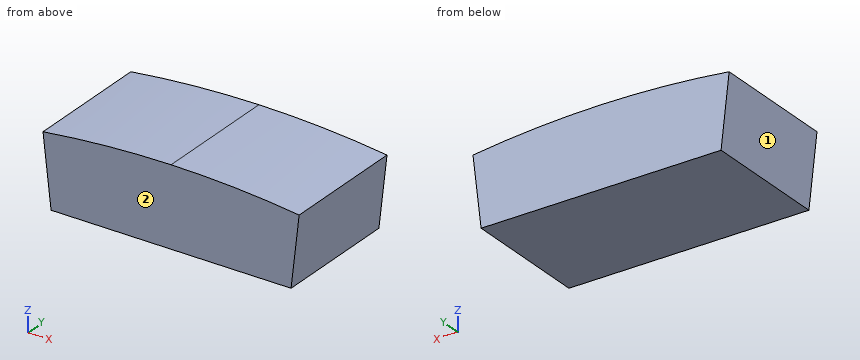
```python
from build123d import *

# Parameters (mm, degrees)
F1_DEPTH = 78.8


with BuildPart() as f1:
    # F0 (on Front) → F1 (new body)
    with BuildSketch(Plane.XZ):
        with BuildLine():
            Line((-62.92016, 6.494325), (-57.92016, -37.305675))
            Line((-57.92016, -37.305675), (90.57984, -37.305675))
            Line((90.57984, -37.305675), (95.57984, 6.494325))
            ThreePointArc((95.57984, 6.494325), (56.033626, 10.243084), (16.32984, 11.494325))
            ThreePointArc((16.32984, 11.494325), (-23.373946, 10.243084), (-62.92016, 6.494325))
        make_face()
    extrude(amount=F1_DEPTH)


solid = f1.part
```
The listing builds one solid part. Answer for the finished solid, in the listing's coordinates (mm). Face numbers are marked on the shaded views. Coordinates: 2 decimals unless noted, no trailing zeros. Write each loop counter-clockwise with the first axis right and the second up, starting at its lowest first coordinate (ties: lowest second). Pieces come first, ordered by that corner, then holes. Notation, with made-up numbers: M 76.25,-1 L 89.25,-1 A23 ccw 89.25,12 Z; hole C 66,53 d3. An arc over 180 degrees is marked long. Use a Markdown table: item, result. Add a question column.
1. Given P1, Ø8, axis at x = -43.5, y = -55, coming from the +Z side; P2, Ø10, axis at x = -23.5, y = -35.5, coming from the +Z side, each flat-ended and moving along its own axis, determine where each tip first touches the part or whether it passes through.
2. Section C-C (z = -21) is taken. Give the vertices of the cut face in (x, y), plus the area to 3 significant figures.
3. Straight lines are drawn through the part: line 1 along Z through (x, y) = (18.5, -48); line 2 along X through (y, z) = (-31, -8); line 3 along Z through (x, y) = (80, -9). For each, find the intervals that lie inside material, in ascending order. Write a range as [from, to].
4. For a pull along Z with two mould halves and no side action, classify the marked faces 1 and 2 as +Z half, -Z half, draft (parallel to the pull), parting line (faces both ways), or undercut.
5. Section B-B (x = -28.5) is taken. Give the vertices of the cut face in (y, z), plus the area to 3 significant figures.
6. Section A-A (y = -18) is taken. Give the vertices of the cut face in (x, z), plus the area to 3 significant figures.
Data:
| question | item | result |
|---|---|---|
| 1 | P1 | stops at z = 9.02 |
| 1 | P2 | stops at z = 10.53 |
| 2 | outline | M -59.78,-78.8 L 92.44,-78.8 L 92.44,0 L -59.78,0 Z |
| 2 | area | 12,000 mm2 |
| 3 | line 1 | z = [-37.31, 11.49] |
| 3 | line 2 | x = [-61.27, 93.93] |
| 3 | line 3 | z = [-37.31, 8.27] |
| 4 | face 1 | -Z half |
| 4 | face 2 | draft |
| 5 | outline | M -78.8,-37.31 L 0,-37.31 L 0,9.9 L -78.8,9.9 Z |
| 5 | area | 3,720 mm2 |
| 6 | outline | M -62.92,6.49 L -57.92,-37.31 L 90.58,-37.31 L 95.58,6.49 A630.56 ccw 16.33,11.49 A630.56 ccw Z |
| 6 | area | 7,250 mm2 |
